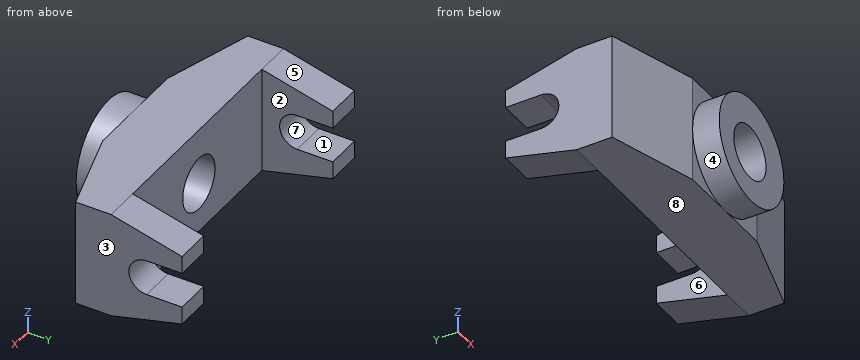
Autodesk Inventor part; units mm, degrees
ref_plane "YZ Plane" through (0, 0, 0) normal (1, 0, 0) x (0, 1, 0)
ref_plane "XZ Plane" through (0, 0, 0) normal (0, 1, 0) x (-1, 0, 0)
ref_plane "XY Plane" through (0, 0, 0) normal (0, 0, 1) x (1, 0, 0)
sketch "Sketch1" plane through (0, 0, 0) normal (0, 0, 1) x (1, 0, 0)
  line L0 (0, 0) -> (0, 25.4)
  line L1 (0, 25.4) -> (-203.2, 25.4)
  line L2 (-203.2, 25.4) -> (-203.2, 0)
  line L3 (-203.2, 0) -> (-139.7, -19.05)
  line L4 (-139.7, -19.05) -> (-63.5, -19.05)
  line L5 (-63.5, -19.05) -> (0, 0)
  dimension "d0" = 203.2
  dimension "d1" = 25.4
  dimension "d2" = 63.5
  dimension "d3" = 44.45
extrude "Extrusion1" add sketch "Sketch1" against normal blind 76.2
sketch "Sketch2" plane through (0, 0, 0) normal (1, 0, 0) x (0, 0, -1)
  line L0 (12.7, 76.2) -> (25.4, 76.2)
  line L1 (25.4, 76.2) -> (25.4, 50.8)
  line L2 (76.2, 25.4) -> (63.5, 76.2)
  line L3 (63.5, 76.2) -> (50.8, 76.2)
  line L4 (0, 25.4) -> (76.2, 25.4)
  line L5 (50.8, 76.2) -> (50.8, 50.8)
  arc A0 (25.4, 50.8) -> (50.8, 50.8) centre (38.1, 50.8) ccw
  line L6 (0, 25.4) -> (12.7, 76.2)
  line L7 (0, 25.4) -> (76.2, 25.4)
  point P0 (0, 0)
  dimension "d6" = 12.7
  dimension "d7" = 25.4
  dimension "d8" = 76.2
  dimension "d9" = 76.2
  dimension "d10" = 50.8
extrude "Extrusion2" add sketch "Sketch2" against normal blind 203.2
sketch "Sketch3" plane through (0, 76.2, -12.7) normal (0, 1, 0) x (1, 0, 0)
  line L0 (0, -12.7) -> (-203.2, -12.7)
  line L1 (-177.8, -12.7) -> (-177.8, 63.5)
  line L2 (-139.7, 63.5) -> (-203.2, 63.5)
  line L3 (-177.8, -12.7) -> (-25.4, -12.7)
  line L4 (-63.5, -12.7) -> (0, -12.7)
  line L5 (-25.4, -12.7) -> (-25.4, 63.5)
  line L6 (0, 63.5) -> (-63.5, 63.5)
  line L7 (-25.4, 63.5) -> (-177.8, 63.5)
  line L8 (-203.2, 12.7) -> (-203.2, 38.1)
  line L9 (0, 38.1) -> (0, 12.7)
  dimension "d13" = 25.4
  dimension "d14" = 25.4
extrude "Extrusion3" cut sketch "Sketch3" against normal blind 50.8
sketch "Sketch4" plane through (-139.7, -19.05, 0) normal (0, -1, 0) x (1, 0, 0)
  circle A0 centre (38.1, -38.1) radius 38.1
  line L0 (0, 0) -> (76.2, 0)
  line L1 (76.2, 0) -> (76.2, -76.2)
  point P0 (139.7, 0)
  dimension "d17" = 76.2
extrude "Extrusion4" add sketch "Sketch4" along normal blind 19.05 contours A0
hole "Hole1" at (-103.5367, -38.1, -40.3531) direction (0, 1, 0) diameter 38.1 end through all
properties part number "HW 7 Part 1" material "Iron, Cast"
Work out the finished part from the listing and answer in its coordinate system (mm). Face numbers are marked on the shaded views. A direction names the side the tool comes from. Round coordinates to 2 decimals unless told otherwise and drop trailing zeros. Order: outer loops, then holes, each group sorted by start corner. A loop starts at its lowest first (then second) coordinate and runs counter-clockwise, first axis right, second up.
Q1. Given pin 1 Ø4 at (x, z) = (-119.5, -43.5) entering from -Y; pin 2 Ø12 at (x, z) = (-80.5, -26.5) entering from +Y; pin 3 Ø12.5 at (x, y) = (-194, 58) entering from +Z; pin 4 Ø6 at (x, z) = (-33, -36) entering from -Y, each flat-ended and moving along its own axis, determine where each tip first touches the part or whether it passes through.
Solution:
pin 1: passes through
pin 2: stops at y = 25.4
pin 3: stops at z = -6.59
pin 4: stops at y = -10.8
Q2. A cutting plane is placed at B-B, the plane x = -189.5. Determine the outline of the cut face in (y, z), then the cut area to 3 significant figures.
Solution:
outline: (-4.11, -76.2) - (25.4, -76.2) - (76.2, -63.5) - (76.2, -50.8) - (50.8, -50.8) arc R12.7 cw to (50.8, -25.4) - (76.2, -25.4) - (76.2, -12.7) - (25.4, 0) - (-4.11, 0) - close
area: 4,580 mm2
Q3. The mould has two halves that part along Z. Classify the marked faces 6, 7 and 8: pulls with the +Z half, pulls with the -Z half, needs draft (parallel to the pull), parting line crosses it, or undercut.
Solution:
face 6: needs draft
face 7: undercut
face 8: pulls with the -Z half
Q4. A tool of negligible diameter and unlimited length cuts with its end or side. For the marked faces 1, 2, 3, 4 and 5, from which of +Z, -Z, +X, -X, +Y, -Y can it reach the whole face along a straight path? Write none if from no direction.
Solution:
face 1: +X, -X, +Y
face 2: +Z, -Z, +Y
face 3: +Z, -Z, +X, +Y, -Y
face 4: -Y
face 5: +Z, +X, -X, +Y
Q5. A cutting plane is placed at D-D, the plane y = -12.5. Determine the outline of the cut face in (x, z), then the cut area to 3 significant figures.
Solution:
outline: (-161.53, -76.2) - (-41.67, -76.2) - (-41.67, 0) - (-161.53, 0) - close; hole circle Ø38.1 at (-103.54, -40.35)
area: 7,990 mm2
Q6. A cutting plane is placed at C-C, the plane x = -114.5. Determine the outline of the cut face in (y, z).
Solution:
outline: (-38.1, -73.95) - (-19.05, -73.95) - (-19.05, -76.2) - (25.4, -76.2) - (25.4, -55.93) - (-38.1, -55.93) - close; (-38.1, -24.77) - (25.4, -24.77) - (25.4, 0) - (-19.05, 0) - (-19.05, -2.25) - (-38.1, -2.25) - close
Q7. Find the intervals of material crossed by line 1 along Z through (x, y) = (-103, -33); line 2 along X through (y, z) = (1.5, -52.5); line 3 along X through (y, z) = (4, -44), in increasing order.
Solution:
line 1: z = -76.17 to -59.4, -21.31 to -0.03
line 2: x = -203.2 to -118.21, -88.86 to 0
line 3: x = -203.2 to -122.23, -84.84 to 0
Q8. A cutting plane is placed at A-A, the plane z = -56. Determine the outline of the cut face in (x, y), then the cut area to 3 significant figures.
Solution:
outline: (-203.2, 0) - (-139.7, -19.05) - (-135.23, -19.05) - (-135.23, -38.1) - (-114.4, -38.1) - (-114.4, 25.4) - (-177.8, 25.4) - (-177.8, 76.2) - (-203.2, 76.2) - close; (-92.67, -38.1) - (-67.97, -38.1) - (-67.97, -19.05) - (-63.5, -19.05) - (0, 0) - (0, 76.2) - (-25.4, 76.2) - (-25.4, 25.4) - (-92.67, 25.4) - close
area: 10,300 mm2
